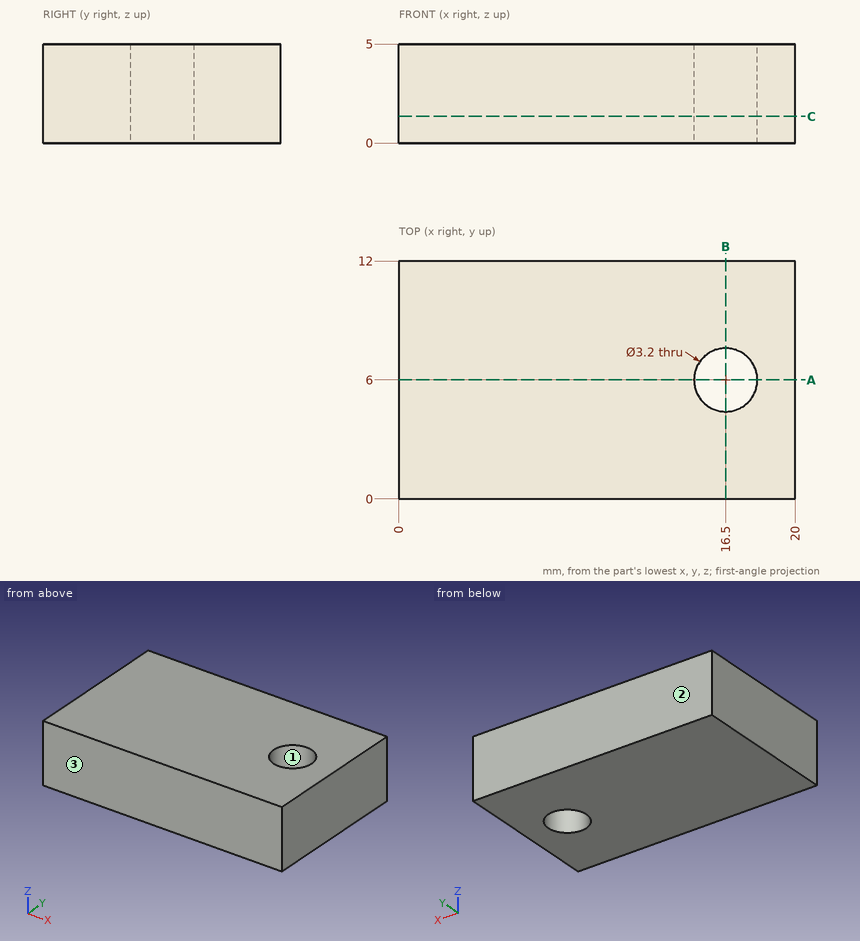
Job drawing, mm, ordinate dimensions from the low corner. One solid piece. Round coordinates to 2 decimals unless told otherwise and drop trailing zeros. Loops run counter-clockwise (first coordinate to the right, second up) from the corner with the lowest first, then second, coordinate; pieces in that order, holes last. Notation, with made-up numbers: (-24.75, 78.25) -> (25.25, 78.25) arc R14 ccw to (25.25, 84.25) -> close; hole circle Ø11 at (62, 49.25). An arc over 180 degrees is marked (long way). Use a Markdown table: item, result.
1) Cut at B-B, the plane x = 16.5. List the corners of the cut face in (y, z).
The answers:
| item | result |
|---|---|
| outline | (0, 0) -> (4.4, 0) -> (4.4, 5) -> (0, 5) -> close; (7.6, 0) -> (12, 0) -> (12, 5) -> (7.6, 5) -> close |
2) Cut at C-C, the plane z = 1.35. List the corners of the cut face in (x, y), and give its area (3 significant figures).
The answers:
| item | result |
|---|---|
| outline | (0, 0) -> (20, 0) -> (20, 12) -> (0, 12) -> close; hole circle Ø3.2 at (16.5, 6) |
| area | 232 mm2 |
3) Pull direction Y, two halves, no side cores. Call the marked faces 1, 2 and 3: pulls with the +Y half, pulls with the -Y half, needs draft (parallel to the pull), parting line crosses it, or undercut.
The answers:
| item | result |
|---|---|
| face 1 | undercut |
| face 2 | pulls with the +Y half |
| face 3 | pulls with the -Y half |
4) Drop a flat-ended pin along its axis: pin 1 Ø3 at (x, y) = (16.5, 6) entering from -Z. Give the stop position or say it passes through.
The answers:
| item | result |
|---|---|
| pin 1 | passes through |
5) Probe line 1 (Y direction, x = 16.5, z = 3.3); line 2 (X direction, y = 6.75, z = 4.15); line 3 (X direction, y = 7, z = 4.65). List the from-to ranges inside material, lowest first. Write a range as [from, to].
The answers:
| item | result |
|---|---|
| line 1 | y = [0, 4.4], [7.6, 12] |
| line 2 | x = [0, 15.09], [17.91, 20] |
| line 3 | x = [0, 15.25], [17.75, 20] |
6) Cut at A-A, the plane y = 6. List the corners of the cut face in (x, z).
The answers:
| item | result |
|---|---|
| outline | (0, 0) -> (14.9, 0) -> (14.9, 5) -> (0, 5) -> close; (18.1, 0) -> (20, 0) -> (20, 5) -> (18.1, 5) -> close |
